Here's how the part is built. I have some questions about the finished solid (model axes, mm). Give positions to 0.01 mm unless a question says otherwise; leave off trailing zeros. Write each loop counter-clockwise with the first axis right and the second up, starting at its lowest first coordinate (ties: lowest second). Pieces come first, ordered by that corner, then holes. Notation, with made-up numbers: (63.5, 58.5) - (104.5, 58.5) arc R16 cw to (104.5, 68.5) - close; hole circle Ø4 at (-1, 43.5). An arc over 180 degrees is marked (long way). Use a Markdown table: item, result.
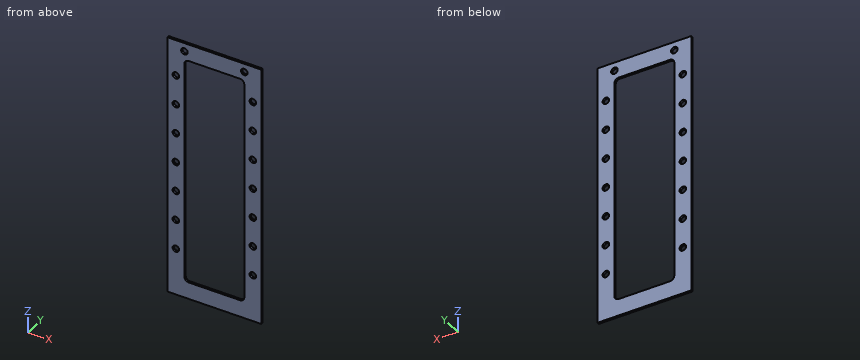
```python
from build123d import *

# Parameters (mm, degrees)
BOSS_EXTRUDE1_DEPTH   = 1.5875
F_8_CLEARANCE_HOLE1_D = 4.9149


with BuildPart() as part:
    # Sketch1 → Boss-Extrude1 (new body)
    with BuildSketch(Plane(origin=(0, 0, 0), x_dir=(1, 0, 0), z_dir=(0, 1, 0))):
        with BuildLine():
            Line((0, 0), (69.85, 0))
            Line((69.85, 0), (69.85, 196.8246))
            ThreePointArc((69.85, 196.8246), (69.842560512, 196.842560512), (69.8246, 196.85))
            Line((69.8246, 196.85), (0.0254, 196.85))
            ThreePointArc((0.0254, 196.85), (0.007439488, 196.842560512), (0, 196.8246))
            Line((0, 196.8246), (0, 0))
        make_face()
        with BuildLine():
            Line((12.7, 15.875), (12.7, 180.975))
            ThreePointArc((12.7, 180.975), (13.62993597, 183.22006403), (15.875, 184.15))
            Line((15.875, 184.15), (53.975, 184.15))
            ThreePointArc((53.975, 184.15), (56.22006403, 183.22006403), (57.15, 180.975))
            Line((57.15, 180.975), (57.15, 15.875))
            ThreePointArc((57.15, 15.875), (56.22006403, 13.62993597), (53.975, 12.7))
            Line((53.975, 12.7), (15.875, 12.7))
            ThreePointArc((15.875, 12.7), (13.62993597, 13.62993597), (12.7, 15.875))
        make_face(mode=Mode.SUBTRACT)
    extrude(amount=BOSS_EXTRUDE1_DEPTH)

    # #8 Clearance Hole1 (through all)
    with Locations(Plane(origin=(0, 0, 0), x_dir=(-1, 0, 0), z_dir=(0, -1, 0))):
        with Locations((-6.35, 161.417), (-57.15, 6.35), (-12.7, 6.35), (-63.5, 27.305), (-6.35, 27.305), (-63.5, 139.065), (-63.5, 116.713), (-63.5, 94.361), (-63.5, 72.009), (-6.35, 49.657), (-6.35, 72.009), (-6.35, 94.361), (-6.35, 116.713), (-6.35, 139.065), (-63.5, 49.657), (-63.5, 161.417)):
            Hole(F_8_CLEARANCE_HOLE1_D / 2)


solid = part.part
```
Item 1: If we section it at A-A, the plane x = 35: Write out the boundary of the cut face in (y, z).
Values:
| item | result |
|---|---|
| outline | (0, -196.85) - (1.59, -196.85) - (1.59, -184.15) - (0, -184.15) - close; (0, -12.7) - (1.59, -12.7) - (1.59, 0) - (0, 0) - close |
Item 2: If we section it at B-B, the plane x = 63.5: Count the separate pieces of the cut face and the enclosed holes in it, plus the area to 3 significant figures.
Values:
| item | result |
|---|---|
| separate pieces | 8 |
| enclosed holes | 0 |
| area | 258 mm2 |
Item 3: Will this pin go through, and if not, where does the flat tip stop? pin 1 Ø3 at (x, z) = (6.35, -94.361) entering from -Y.
Values:
| item | result |
|---|---|
| pin 1 | passes through |
Item 4: If we section it at D-D, the plane z = -6.35: Write out the boundary of the cut face in (x, y).
Values:
| item | result |
|---|---|
| outline | (0, 0) - (10.24, 0) - (10.24, 1.59) - (0, 1.59) - close; (15.16, 0) - (54.69, 0) - (54.69, 1.59) - (15.16, 1.59) - close; (59.61, 0) - (69.85, 0) - (69.85, 1.59) - (59.61, 1.59) - close |
Item 5: If we section it at C-C, the plane z = -175: Write out the boundary of the cut face in (x, y), plus the area to 3 significant figures.
Values:
| item | result |
|---|---|
| outline | (0, 0) - (12.7, 0) - (12.7, 1.59) - (0, 1.59) - close; (57.15, 0) - (69.85, 0) - (69.85, 1.59) - (57.15, 1.59) - close |
| area | 40.3 mm2 |
Item 6: I need wall thicknesses on line 1 along Z through (x, y) = (46, 0.9); line 2 along X through (y, z) = (1.55, -19). Which ranges of each line are inside material? Lowest first, please. Write a range as [from, to].
Values:
| item | result |
|---|---|
| line 1 | z = [-196.85, -184.15], [-12.7, 0] |
| line 2 | x = [0, 12.7], [57.15, 69.85] |
